```python
from build123d import *

# Parameters (mm, degrees)
PAD_DEPTH       = 20
SKETCH001_R     = 1.6
POCKET_DEPTH    = 5.68
SKETCH002_W     = 5
SKETCH002_H     = 5
SKETCH002_R     = 1.6
PAD001_DEPTH    = 1
SKETCH003_R     = 1.6
POCKET001_DEPTH = 2.4
SKETCH004_W     = 5.88
SKETCH004_H     = 2.68
POCKET002_DEPTH = 20.001


with BuildPart() as part:
    # Sketch → Pad (new body)
    with BuildSketch(Plane.XY):
        Polygon((2.94, -2.84), (-2.94, -2.84), (-5.44, -0.52), (-5.44, 1.16), (-2.94, 1.16), (-2.94, 2.84), (2.94, 2.84), (2.94, 1.16), (5.44, 1.16), (5.44, -0.52), align=None)
    extrude(amount=PAD_DEPTH)

    # Sketch001 (on Face6 of Pad) → Pocket (cut)
    with BuildSketch(Plane(origin=(0, 2.84, 0), x_dir=(-1, 0, 0), z_dir=(0, 1, 0))):
        with Locations((0, 10)):
            Circle(SKETCH001_R)
    extrude(amount=-POCKET_DEPTH, mode=Mode.SUBTRACT)

    # Sketch002 (on Face11 of Pocket) → Pad001 (join)
    with BuildSketch(Plane(origin=(0, 2.84, 0), x_dir=(-1, 0, 0), z_dir=(0, 1, 0))):
        with Locations((0, 10)):
            Rectangle(SKETCH002_W, SKETCH002_H)
        with Locations((0, 10)):
            Circle(SKETCH002_R, mode=Mode.SUBTRACT)
    extrude(amount=PAD001_DEPTH)

    # Sketch003 (on Face1 of Pad001) → Pocket001 (cut)
    with BuildSketch(Plane.XZ.offset(2.84)):
        Polygon((0, 6.686009), (2.87, 8.343005), (2.87, 11.656995), (0, 13.313991), (-2.87, 11.656995), (-2.87, 8.343005), align=None)
        with Locations((0, 10)):
            Circle(SKETCH003_R, mode=Mode.SUBTRACT)
    extrude(amount=-POCKET001_DEPTH, mode=Mode.SUBTRACT)

    # Sketch004 (on Face3 of Pocket001) → Pocket002 (cut, through all)
    with BuildSketch(Plane(origin=(0, 0, 0), x_dir=(1, 0, 0), z_dir=(0, 0, -1))):
        with Locations((0, -2.5)):
            Rectangle(SKETCH004_W, SKETCH004_H)
    extrude(amount=-POCKET002_DEPTH, mode=Mode.SUBTRACT)


solid = part.part
```
Model file for the job. Use its own axes, mm. A direction names the side the tool comes from. Coordinates: 2 decimals unless noted, no trailing zeros. Order: outer loops, then holes, each group sorted by start corner. A loop starts at its lowest first (then second) coordinate and runs counter-clockwise, first axis right, second up. Notation, with made-up numbers: (-6.5, 59.5) - (41.5, 59.5) arc R21 cw to (41.5, 85.5) - close; hole circle Ø4 at (-33.75, 18.25). An arc over 180 degrees is marked (long way). Return JSON: item names as keys, results as strings. Group by question number.
1) Saw through at D-D, the plane z = 16.5. Write the cut outline in (x, y), plus the area to 3 significant figures.
2) Flat gauge pin, fed straight in: P1, Ø0.7, axis at y = -2, z = 9.5, coming from the -X side. Where does the tip first touch, or does it go through?
3) Saw through at B-B, the plane y = 0.2. Write the cut outline in (x, z).
4) Saw through at A-A, the plane z = 10. Write the cut outline in (x, y), plus the area to 3 significant figures.
5) Mould opens along Z. For faces 1 (the flat face through (-1.46, -1.66, 7.53)), 2 (the flat face through (0, -1, 0)), 3 (the flat face through (-5.44, 0, 10)), 4 (the flat face through (0, -1, 20)) say: released by +Z, released by -Z, zero draft, split by the parting line, or undercut.
6) Probe line 1 (X direction, y = 0.75, z = 10); line 2 (Z direction, x = 0, y = 0.75); line 3 (X direction, y = -2.35, z = 11.75). List the from-to ranges inside material, lowest first. Write a range as from..to.
7) Saw through at C-C, the plane x = 2.5. Write the cut outline in (y, z).
8) Tool access for faces 5 (the flat face through (1.46, -1.66, 12.47)), 6 (the flat face through (5.44, 0, 10)): list every direction of +Z, -Z, +X, -X, +Y, -Y with a clear straight run to the whole face (end or side of a thin tool).
Values found:
{
 "1": {"outline": "(-5.44, -0.52) - (-2.94, -2.84) - (2.94, -2.84) - (5.44, -0.52) - (5.44, 1.16) - (-5.44, 1.16) - close", "area": "37.7 mm²"},
 "2": {"P1": "stops at x = -4.22"},
 "3": {"outline": "(-5.44, 0) - (5.44, 0) - (5.44, 20) - (-5.44, 20) - close; hole circle Ø3.2 at (0, 10)"},
 "4": {"outline": "(-5.44, -0.52) - (-2.94, -2.84) - (-2.87, -2.84) - (-2.87, -0.44) - (-1.6, -0.44) - (-1.6, 1.16) - (-5.44, 1.16) - close; (1.6, -0.44) - (2.87, -0.44) - (2.87, -2.84) - (2.94, -2.84) - (5.44, -0.52) - (5.44, 1.16) - (1.6, 1.16) - close", "area": "18.8 mm²"},
 "5": {"face 1": "undercut", "face 2": "released by -Z", "face 3": "zero draft", "face 4": "released by +Z"},
 "6": {"line 1": "x = -5.44..-1.6, 1.6..5.44", "line 2": "z = 0..8.4, 11.6..20", "line 3": "x = -3.47..-2.71, 2.71..3.47"},
 "7": {"outline": "(-2.84, 0) - (1.16, 0) - (1.16, 20) - (-2.84, 20) - (-2.84, 11.87) - (-0.44, 11.87) - (-0.44, 8.13) - (-2.84, 8.13) - close"},
 "8": {"face 5": "-Y", "face 6": "+Z, -Z, +X, +Y, -Y"}
}
